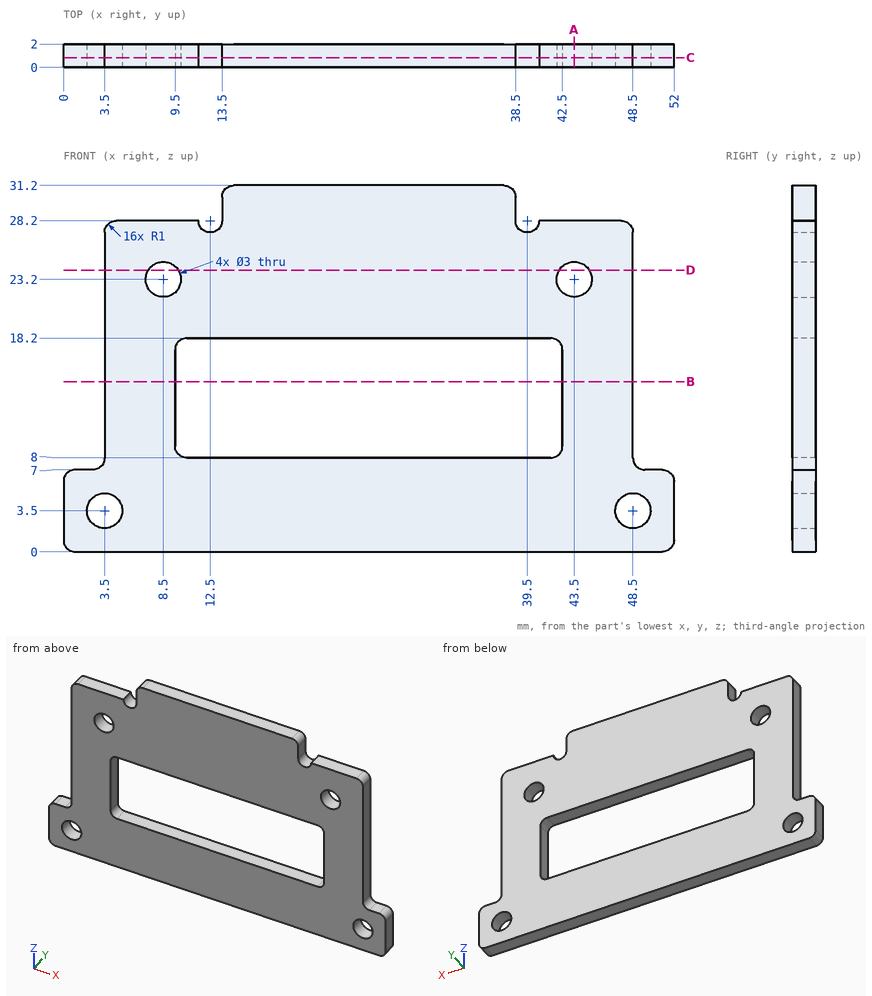
Source: three-view drawing plus pictorial views. Frame: mm from the lowest corner of the part. Round coordinates to 2 decimals unless told otherwise and drop trailing zeros. Loops run counter-clockwise (first coordinate to the right, second up) from the corner with the lowest first, then second, coordinate; pieces in that order, holes last.
Q1. Section D-D on z = 24. Return loops of the section in (x, y), plus the area to 3 significant figures.
Q2. Pin query (flat end, axial travel): P1, Ø0.6, axis at y = 0.5, z = 29.5, coming from the -X side; P2, Ø1.2, axis at x = 1.5, y = 1, coming from the +Z side; P3, Ø1, axis at y = 1, z = 12, coming from the +X side. Return the tip coordinate at first contact, or that it passes through.
Q3. Section B-B on z = 14.5. Return loops of the section in (x, y).
Q4. Section C-C on y = 0.85. State how many separate pieces and enclosed holes the cut face has, plus the area to 3 significant figures.
Q5. Section A-A on x = 43.5. Return loops of the section in (y, z), plus the area to 3 significant figures.
Q6. Material intervals for L1, parallel to X at y = 0.55, z = 23.2; L2, parallel to Z at x = 43.5, y = 1.05; L3, parallel to Z at x = 24, y = 1.35, sorted ascending.
Evaluation:
1. outline: (3.5, 0) - (7.23, 0) - (7.23, 2) - (3.5, 2) - close; (9.77, 0) - (42.23, 0) - (42.23, 2) - (9.77, 2) - close; (44.77, 0) - (48.5, 0) - (48.5, 2) - (44.77, 2) - close
1. area: 79.8 mm2
2. P1: stops at x = 13.5
2. P2: stops at z = 7
2. P3: stops at x = 48.5
3. outline: (3.5, 0) - (9.5, 0) - (9.5, 2) - (3.5, 2) - close; (42.5, 0) - (48.5, 0) - (48.5, 2) - (42.5, 2) - close
4. separate pieces: 1
4. enclosed holes: 5
4. area: 1,020 mm2
5. outline: (0, 0) - (2, 0) - (2, 21.7) - (0, 21.7) - close; (0, 24.7) - (2, 24.7) - (2, 28.2) - (0, 28.2) - close
5. area: 50.4 mm2
6. L1: x = 3.5 to 7, 10 to 42, 45 to 48.5
6. L2: z = 0 to 21.7, 24.7 to 28.2
6. L3: z = 0 to 8, 18.2 to 31.2
